Job drawing, mm, ordinate dimensions from the low corner. One solid piece. Give positions to 0.01 mm unless a question says otherwise; leave off trailing zeros. Write each loop counter-clockwise with the first axis right and the second up, starting at its lowest first coordinate (ties: lowest second). Pieces come first, ordered by that corner, then holes. Notation, with made-up numbers: M 22.5,88.5 L 81.5,88.5 A11 cw 81.5,100.5 Z; hole C 54,-2 d6. An arc over 180 degrees is marked long. Answer as CSV lines item,"result". Start each with the question number.
1) Slice it at A-A, the plane x = 6. Give the cut face in (y, z), plus the area to 3 significant figures.
2) Slice it at C-C, the plane z = 67.5. Give the cut face in (x, y), plus the area to 3 significant figures.
3) Wall check: line 1 along Z through (x, y) = (14, 4.5); line 2 along X through (y, z) = (0.25, 70). Give the ranges that are in metal, low to high. Write a range as from..to.
4) Slice it at B-B, the plane y = 2.75. Give the cut face in (x, z).
5) Pin check, flat tips, straight feed: pin 1 Ø12 at (x, z) = (38, 37.5) entering from -Y; pin 2 Ø1 at (y, z) = (3.5, 64) entering from -X. Stop position of each tip, or through.
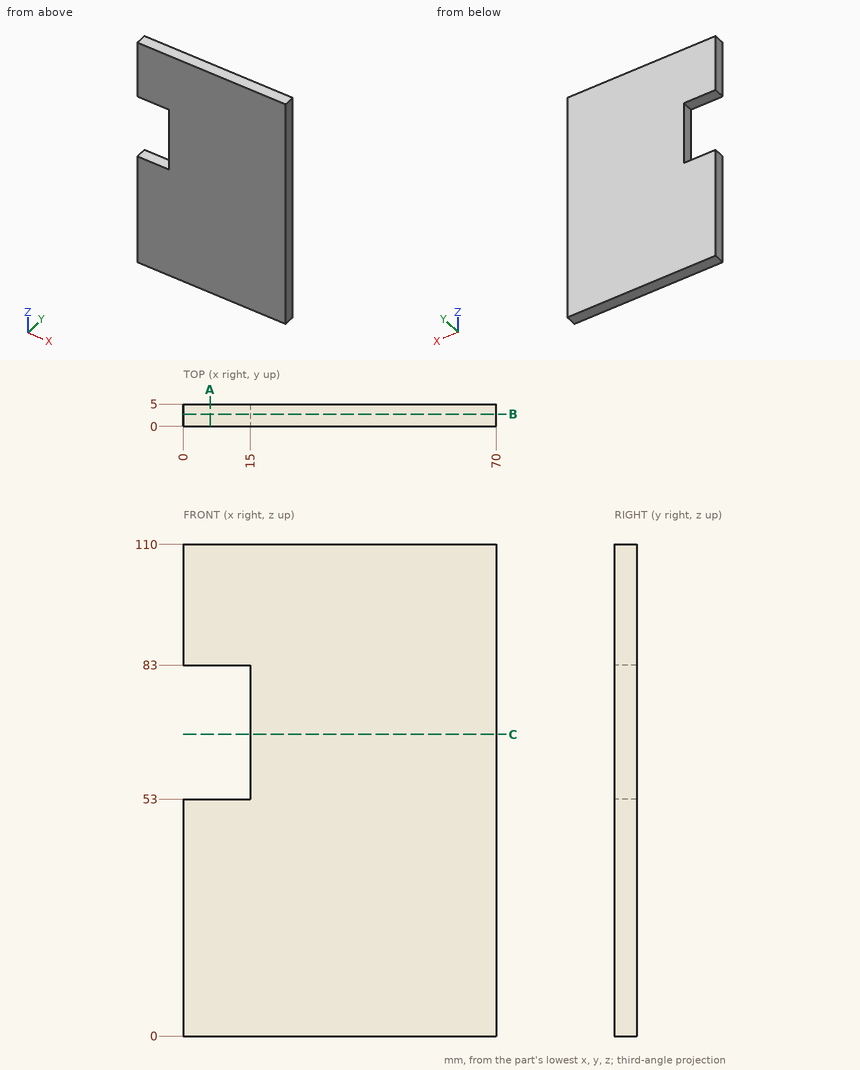
Found:
1,outline,"M 0,0 L 5,0 L 5,53 L 0,53 Z; M 0,83 L 5,83 L 5,110 L 0,110 Z"
1,area,"400 mm²"
2,outline,"M 15,0 L 70,0 L 70,5 L 15,5 Z"
2,area,"275 mm²"
3,line 1,"0..53, 83..110"
3,line 2,"15..70"
4,outline,"M 0,0 L 70,0 L 70,110 L 0,110 L 0,83 L 15,83 L 15,53 L 0,53 Z"
5,pin 1,"y = 0"
5,pin 2,"x = 15"
